Part model, mm, in its own coordinate system. Face numbers are marked on the shaded views. A direction names the side the tool comes from. Coordinates: 2 decimals unless noted, no trailing zeros. Write each loop counter-clockwise with the first axis right and the second up, starting at its lowest first coordinate (ties: lowest second). Pieces come first, ordered by that corner, then holes. Notation, with made-up numbers: (61.5, -23) - (109.5, -23) arc R25 cw to (109.5, 1) - close; hole circle Ø6 at (79, 28). An arc over 180 degrees is marked (long way). Use a Markdown table: item, result.
```python
from build123d import *

# Parameters (mm, degrees)
SKETCH_1_W          = 72
SKETCH_1_H          = 72
EXTRUDE_1_DEPTH     = 44.5
SKETCH_4_R          = 2.5
SKETCH_4_W          = 10
SKETCH_4_H          = 15
SKETCH_4_W_2        = 6
SKETCH_4_H_2        = 13
CUT_EXTRUDE_2_DEPTH = 10
FILLET_1_R          = 5
SKETCH_2_R          = 1.05
CUT_EXTRUDE_1_DEPTH = 5
SKETCH_3_R          = 4
SKETCH_3_R_2        = 2.25
EXTRUDE_2_DEPTH     = 1


with BuildPart() as part:
    # 草图1 → 凸台-拉伸1 (new body)
    with BuildSketch(Plane.XY):
        Rectangle(SKETCH_1_W, SKETCH_1_H)
    extrude(amount=EXTRUDE_1_DEPTH)

    # 草图4 → 切除-拉伸2 (cut)
    with BuildSketch(Plane.ZY.offset(36)):
        with Locations((10, 22.5)):
            Circle(SKETCH_4_R)
        with Locations((9, 3.5)):
            Rectangle(SKETCH_4_W, SKETCH_4_H)
        Polygon((18, -11), (18, -26), (21, -26), (23.826446608, -23.5), (23.826446608, -13.5), (21, -11), align=None)
        with Locations((8, -19.5)):
            Rectangle(SKETCH_4_W_2, SKETCH_4_H_2)
        Polygon((18, 10.5), (18, -4.5), (21, -4.5), (23.826446608, -2), (23.826446608, 8), (21, 10.5), align=None)
    extrude(amount=-CUT_EXTRUDE_2_DEPTH, mode=Mode.SUBTRACT)

    # 圆角1
    fillet_1_edges = [part.edges().sort_by_distance(p)[0] for p in [
        (36, -36, 22.25),
        (-36, -36, 22.25),
        (-36, 36, 22.25),
        (36, 36, 22.25),
    ]]
    fillet(fillet_1_edges, radius=FILLET_1_R)

    # 草图2 → 切除-拉伸1 (cut)
    with BuildSketch(Plane(origin=(0, 0, 0), x_dir=(-1, 0, 0), z_dir=(0, 0, -1))):
        with Locations((0, 27.5)):
            Circle(SKETCH_2_R)
        with Locations((0, -27.5)):
            Circle(SKETCH_2_R)
    extrude(amount=-CUT_EXTRUDE_1_DEPTH, mode=Mode.SUBTRACT)

    # 草图3 → 凸台-拉伸2 (add)
    # profile 1 of 4: a face of its own
    with BuildSketch(Plane(origin=(0, 0, 0), x_dir=(-1, 0, 0), z_dir=(0, 0, -1))):
        with Locations(Location((29.5, -29.5, 0), (0, 0, 180))):
            Circle(SKETCH_3_R)
        with Locations((29.5, -29.5)):
            Circle(SKETCH_3_R_2, mode=Mode.SUBTRACT)
    # profile 2 of 4: a face of its own
    with BuildSketch(Plane(origin=(0, 0, 0), x_dir=(-1, 0, 0), z_dir=(0, 0, -1))):
        with Locations(Location((-29.5, -29.5, 0), (0, 0, 180))):
            Circle(SKETCH_3_R)
        with Locations((-29.5, -29.5)):
            Circle(SKETCH_3_R_2, mode=Mode.SUBTRACT)
    # profile 3 of 4: a face of its own
    with BuildSketch(Plane(origin=(0, 0, 0), x_dir=(-1, 0, 0), z_dir=(0, 0, -1))):
        with Locations(Location((-29.5, 29.5, 0), (0, 0, 180))):
            Circle(SKETCH_3_R)
        with Locations((-29.5, 29.5)):
            Circle(SKETCH_3_R_2, mode=Mode.SUBTRACT)
    # profile 4 of 4: a face of its own
    with BuildSketch(Plane(origin=(0, 0, 0), x_dir=(-1, 0, 0), z_dir=(0, 0, -1))):
        with Locations(Location((29.5, 29.5, 0), (0, 0, 180))):
            Circle(SKETCH_3_R)
        with Locations((29.5, 29.5)):
            Circle(SKETCH_3_R_2, mode=Mode.SUBTRACT)
    extrude(amount=EXTRUDE_2_DEPTH)


solid = part.part
```
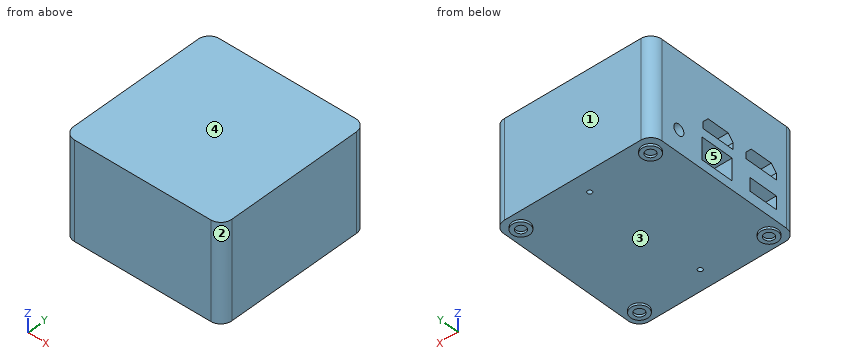
Item 1: Drop flat-ended pins along their axis: P1, Ø1.7, axis at x = 0, y = -27.5, coming from the -Z side; P2, Ø8, axis at x = -29.5, y = 2, coming from the -Z side; P3, Ø5, axis at x = -30.5, y = 29, coming from the -Z side; P4, Ø0.9, axis at x = -32.5, z = 19, coming from the -Y side. Give the stop position or say it passes through.
From the geometry:
| item | result |
|---|---|
| P1 | z = 5 |
| P2 | z = 0 |
| P3 | z = -1 |
| P4 | y = -35.89 |
Item 2: Which spindle directions (+Z, -Z, +X, -X, +Y, -Y) get a long thin tool onto all of the face, cutting with end or side? Do the marked faces 4 and 5. Say none if no direction does.
From the geometry:
| item | result |
|---|---|
| face 4 | +Z, +X, -X, +Y, -Y |
| face 5 | -X |
Item 3: Band-saw the part on C-C, the plane y = 22.5. Give the cut face in (x, z).
From the geometry:
| item | result |
|---|---|
| outline | (-36, 0) - (36, 0) - (36, 44.5) - (-36, 44.5) - (-36, 12.5) - (-26, 12.5) - (-26, 7.5) - (-36, 7.5) - close |
Item 4: Two-plate mould, pull along X, no slides. Class the marked faces 1, 2 and 3: pulls with the +X half, pulls with the -X half, needs draft (parallel to the pull), parting line crosses it, or undercut.
From the geometry:
| item | result |
|---|---|
| face 1 | needs draft |
| face 2 | pulls with the +X half |
| face 3 | undercut |
Item 5: Band-saw the part on D-D, the plane x = 0. Give the cut face in (y, z), then the cut area to 3 significant figures.
From the geometry:
| item | result |
|---|---|
| outline | (-36, 0) - (-28.55, 0) - (-28.55, 5) - (-26.45, 5) - (-26.45, 0) - (26.45, 0) - (26.45, 5) - (28.55, 5) - (28.55, 0) - (36, 0) - (36, 44.5) - (-36, 44.5) - close |
| area | 3,180 mm^2 |
Item 6: Drill centre lines: probe 1 along Y at (x, z) = (0, 3.9); probe 2 along Y at (x, z) = (-29.5, -0.65); probe 3 along Y at (x, z) = (-32, 10). Where is each one in solid material? Low to high.
From the geometry:
| item | result |
|---|---|
| probe 1 | -36 to -28.55, -26.45 to 26.45, 28.55 to 36 |
| probe 2 | -33.5 to -31.75, -27.25 to -25.5, 25.5 to 27.25, 31.75 to 33.5 |
| probe 3 | -35.9 to -26, -13 to -4, 11 to 20, 25 to 35.9 |
Item 7: Band-saw the part on A-A, the plane x = 29.5. Give the cut face in (y, z), then the cut area to 3 significant figures.
From the geometry:
| item | result |
|---|---|
| outline | (-36, 0) - (-33.5, 0) - (-33.5, -1) - (-31.75, -1) - (-31.75, 0) - (-27.25, 0) - (-27.25, -1) - (-25.5, -1) - (-25.5, 0) - (25.5, 0) - (25.5, -1) - (27.25, -1) - (27.25, 0) - (31.75, 0) - (31.75, -1) - (33.5, -1) - (33.5, 0) - (36, 0) - (36, 44.5) - (-36, 44.5) - close |
| area | 3,210 mm^2 |
Item 8: Band-saw the part on B-B, the plane z = 10. Give the cut face in (x, y), then the cut area to 3 significant figures.
From the geometry:
| item | result |
|---|---|
| outline | (-36, -31) arc R5 ccw to (-31, -36) - (31, -36) arc R5 ccw to (36, -31) - (36, 31) arc R5 ccw to (31, 36) - (-31, 36) arc R5 ccw to (-36, 31) - (-36, 25) - (-26, 25) - (-26, 20) - (-36, 20) - (-36, 11) - (-26, 11) - (-26, -4) - (-36, -4) - (-36, -13) - (-26, -13) - (-26, -26) - (-36, -26) - close |
| area | 4,830 mm^2 |
